Autodesk Inventor part; units mm, degrees
ref_plane "YZ Plane" through (0, 0, 0) normal (1, 0, 0) x (0, 1, 0)
ref_plane "XZ Plane" through (0, 0, 0) normal (0, 1, 0) x (-1, 0, 0)
ref_plane "XY Plane" through (0, 0, 0) normal (0, 0, 1) x (1, 0, 0)
sketch "スケッチ1" plane through (0, 0, 0) normal (0, 0, 1) x (1, 0, 0)
  line L0 (-18, 18) -> (18, 18)
  line L1 (18, 18) -> (18, -18)
  line L2 (18, -18) -> (-18, -18)
  line L3 (-18, -18) -> (-18, 18)
  line L4 (-18, 18) -> (18, -18) construction
  line L5 (18, 18) -> (-18, -18) construction
  line L6 (-20, 20) -> (20, 20)
  line L7 (20, 20) -> (20, -20)
  line L8 (20, -20) -> (-20, -20)
  line L9 (-20, -20) -> (-20, 20)
  line L10 (-20, 20) -> (20, -20) construction
  line L11 (20, 20) -> (-20, -20) construction
  point P0 (0, 0)
  dimension "d0" = 36
  dimension "d1" = 36
  dimension "d2" = 40
  dimension "d3" = 40
extrude "押し出し1" add sketch "スケッチ1" along normal blind 39.5
sketch "スケッチ2" plane through (20, -20, 0) normal (1, 0, 0) x (0, 0, -1)
  line L0 (0, 40) -> (-39.5, 40)
  line L1 (0, 40) -> (0, 0)
  line L2 (-39.5, 0) -> (-39.5, 40)
  point P0 (0, 20)
  point P1 (-13, 20)
  point P2 (-26.5, 20)
  dimension "d13" = 13.5
  dimension "d14" = 20
  dimension "d15" = 13
  dimension "d16" = 13
  dimension "d17" = 20
hole "穴1" at (20, 0, 13) at (20, 0, 26.5) direction (-1, 0, 0) diameter 6 end through all
properties part number "Square pipe" material "アルミニウム 6061"
Input: part model. Units: mm. Frame: model coordinates. A direction names the side the tool comes from. Coordinates: 2 decimals unless noted, no trailing zeros. Loops run counter-clockwise (first coordinate to the right, second up) from the corner with the lowest first, then second, coordinate; pieces in that order, holes last. Notation, with made-up numbers: (-25, 21) -> (26, 21) arc R21 cw to (26, 46) -> close; hole circle Ø7 at (23, -25). An arc over 180 degrees is marked (long way). Write item = value, one per line. Start each with the question number.
Item 1: Cut plane B-B, the plane x = 15. Return loops of the section in (y, z), plus the area to 3 significant figures.
Item 2: Material intervals for line 1 (X direction, y = -6.5, z = 8); line 2 (Z direction, x = -19.55, y = 0), sorted ascending.
Item 3: Cut plane A-A, the plane y = 0. Return loops of the section in (x, z), plus the area to 3 significant figures.
Item 4: First-contact query: P1, Ø6, axis at x = 13, y = -14.5, coming from the +Z side. Flat tip, straight axial feed; report the tip coordinate or a pass-through.
Item 5: Mould query, pull axis Y, two halves, no side actions, for faces 3 (the face through (0, 20, 19)), 4 (the face through (0, 18, 19)), 5 (the face through (20, 0, 19)). Classes: pulls with the +Y half, pulls with the -Y half, needs draft (parallel to the pull), parting line crosses it, or undercut.
Item 6: Reachability of faces 1 (the face through (-19, -0.1, 29.5)), 2 (the face through (18, 0, 19)) from +Z, -Z, +X, -X, +Y, -Y: full face, straight path, thin tool, end or side. Return the list, or none.
Item 7: Cut plane C-C, the plane z = 13. Return loops of the section in (x, y), plus the area to 3 significant figures.
Ans:
q1.outline = (-20, 0) -> (-18, 0) -> (-18, 39.5) -> (-20, 39.5) -> close; (18, 0) -> (20, 0) -> (20, 39.5) -> (18, 39.5) -> close
q1.area = 158 mm²
q2.line_1 = -20 to -18, 18 to 20
q2.line_2 = 0 to 10, 16 to 23.5, 29.5 to 39.5
q3.outline = (-20, 0) -> (-18, 0) -> (-18, 10) -> (-20, 10) -> close; (-20, 16) -> (-18, 16) -> (-18, 23.5) -> (-20, 23.5) -> close; (-20, 29.5) -> (-18, 29.5) -> (-18, 39.5) -> (-20, 39.5) -> close; (18, 0) -> (20, 0) -> (20, 10) -> (18, 10) -> close; (18, 16) -> (20, 16) -> (20, 23.5) -> (18, 23.5) -> close; (18, 29.5) -> (20, 29.5) -> (20, 39.5) -> (18, 39.5) -> close
q3.area = 110 mm²
q4.P1 = through
q5.face_3 = pulls with the +Y half
q5.face_4 = undercut
q5.face_5 = needs draft
q6.face_1 = +X, -X
q6.face_2 = +Z, -Z
q7.outline = (-20, -20) -> (20, -20) -> (20, -3) -> (18, -3) -> (18, -18) -> (-18, -18) -> (-18, -3) -> (-20, -3) -> close; (-20, 3) -> (-18, 3) -> (-18, 18) -> (18, 18) -> (18, 3) -> (20, 3) -> (20, 20) -> (-20, 20) -> close
q7.area = 280 mm²
